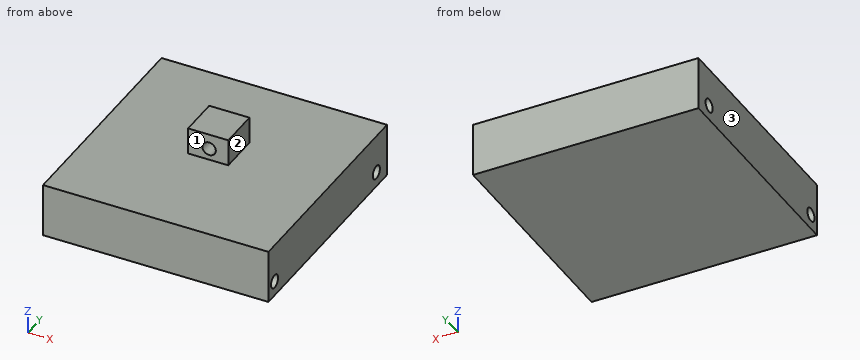
from build123d import *

# Parameters (mm, degrees)
F0_W     = 106.6800057888
F0_H     = 106.6800057888
F1_DEPTH = 25.4
F3_D     = 6.35
F4_W     = 19.0191436559
F4_H     = 19.0191436559
F5_DEPTH = 12.7
F7_D     = 6.35
F7_DEPTH = 7.62
F7_TIP   = 1.9077324654


with BuildPart() as f1:
    # F0 (on Top) → F1 (new body)
    with BuildSketch(Plane.XY):
        with Locations((10.4977674782, 4.2558498681)):
            Rectangle(F0_W, F0_H)
    extrude(amount=F1_DEPTH)

    # F3 (through all)
    with Locations(Plane.YZ.offset(63.8377703726)):
        with Locations((-43.6188168824, 7.1031823754), (48.0126738548, 7.1031823754)):
            Hole(F3_D / 2)

    # F4 (on face) → F5 (join)
    with BuildSketch(Plane.XY.offset(25.4)):
        with Locations((9.5095718279, 9.5095718279)):
            Rectangle(F4_W, F4_H)
    extrude(amount=F5_DEPTH)

    # F7
    with Locations(Plane.XZ):
        with Locations((9.9399928004, 30.9258513153)):
            Hole(F7_D / 2, depth=F7_DEPTH)
            with Locations((0, 0, -(F7_DEPTH + F7_TIP / 2))):  # 118° drill point
                Cone(0, F7_D / 2, F7_TIP, mode=Mode.SUBTRACT)


solid = f1.part
The listing builds one solid part. Answer for the finished solid, in the listing's coordinates (mm). Face numbers are marked on the shaded views. A direction names the side the tool comes from. Round coordinates to 2 decimals unless told otherwise and drop trailing zeros. Order: outer loops, then holes, each group sorted by start corner. A loop starts at its lowest first (then second) coordinate and runs counter-clockwise, first axis right, second up. Notation, with made-up numbers: M 59.25,6.25 L 73.25,6.25 A22 cw 73.25,19.25 Z; hole C -4.75,70 d3. An arc over 180 degrees is marked long. Answer in a Markdown table with one row per item. Add a question column.
1) Which of the six approach directions +Z, -Z, +X, -X, +Y, -Y give full straight-line access (tool end or side, diameter ignored) to the marked faces 1, 2 and 3?
2) The part is cut by section D-D on x = 32.5. Determine the outline of the cut face in (y, z) (3 decimals), plus the area to 3 significant figures.
3) Consider line 1 along Y through (x, z) = (13, 8.5); line 2 along Z through (x, y) = (58.5, 9.5); line 3 along Z through (x, y) = (34, 50.5). Determine where each line is inside the solid, lowest interval first. Write a range as from..to.
4) The part is cut by section C-C on y = 11.5. Determine the outline of the cut face in (x, z).
5) The part is cut by section B-B on x = 17.5. Determine the outline of the cut face in (y, z) (3 decimals), plus the area to 3 significant figures.
6) The part is cut by section A-A on z = 8.5. Determine the outline of the cut face in (x, y), plus the area to 3 significant figures.
7) Flat-ended cylindrical pins translate along their axes: pin 1 Ø3 at (x, y) = (22.5, -12.5) entering from +Z; pin 2 Ø10 at (x, z) = (13, 34.5) entering from -Y; pin 3 Ø6.5 at (x, z) = (13, 30.5) entering from +Y. Find the tip coordinate at first contact, or state that the pin passes through.
Findings below:
| question | item | result |
|---|---|---|
| 1 | face 1 | +Z, +X, -X, -Y |
| 1 | face 2 | +Z, +X, +Y, -Y |
| 1 | face 3 | +Z, -Z, -X, +Y, -Y |
| 2 | outline | M -49.084,0 L 57.596,0 L 57.596,25.4 L -49.084,25.4 Z; hole C -43.619,7.103 d6.35; hole C 48.013,7.103 d6.35 |
| 2 | area | 2,650 mm² |
| 3 | line 1 | y = -49.08..-46.47, -40.77..45.16, 50.86..57.6 |
| 3 | line 2 | z = 0..25.4 |
| 3 | line 3 | z = 0..5.13, 9.08..25.4 |
| 4 | outline | M -42.84,0 L 63.84,0 L 63.84,25.4 L 19.02,25.4 L 19.02,38.1 L 0,38.1 L 0,25.4 L -42.84,25.4 Z |
| 5 | outline | M -49.084,0 L 57.596,0 L 57.596,25.4 L 19.019,25.4 L 19.019,38.1 L 0,38.1 L 0,25.4 L -49.084,25.4 Z; hole C -43.619,7.103 d6.35; hole C 48.013,7.103 d6.35 |
| 5 | area | 2,890 mm² |
| 6 | outline | M -42.84,-49.08 L 63.84,-49.08 L 63.84,-46.47 L -42.84,-46.47 Z; M -42.84,-40.77 L 63.84,-40.77 L 63.84,45.16 L -42.84,45.16 Z; M -42.84,50.86 L 63.84,50.86 L 63.84,57.6 L -42.84,57.6 Z |
| 6 | area | 10,200 mm² |
| 7 | pin 1 | stops at z = 25.4 |
| 7 | pin 2 | stops at y = 0 |
| 7 | pin 3 | stops at y = 19.02 |
